Geometry: final body of the model. Coordinates: model frame, mm. A direction names the side the tool comes from. Coordinates: 2 decimals unless noted, no trailing zeros. Order: outer loops, then holes, each group sorted by start corner. A loop starts at its lowest first (then second) coordinate and runs counter-clockwise, first axis right, second up. Notation, with made-up numbers: (50.25, 17.5) -> (86.25, 17.5) arc R22 cw to (86.25, 37.5) -> close; hole circle Ø6 at (-39, 63.25). An arc over 180 degrees is marked (long way). Answer in a Markdown table with one row per item. Add a question column.
1) Section query B-B on x = 2.75. Return the cut outline in (y, z), then the cut area to 3 significant figures.
2) Ray query, line 1 (X direction, y = 3.75, z = 0); line 2 (Z direction, x = -0.75, y = 9); line 3 (X direction, y = 6.5, z = 1.5). Return the intervals inside material, ascending. Write a range as from..to.
3) Contact query for flat-ended pins moving along their axis: P1, Ø3.5, axis at x = -1.5, z = 0.5, coming from the +Y side; P2, Ø6, axis at x = -4.5, y = 6.5, coming from the -Z side; P3, Ø3, axis at y = 3, z = 4.5, coming from the +X side. Output: stop coordinate, or through.
4) Set-up query: faces 4 (the face through (-4.1, 4.93, 4.38)), 5 (the face through (-3.417, 6.056, -0.759)). Return all of +Z, -Z, +X, -X, +Y, -Y with unobstructed straight access to the full face (end or side cutting, diameter ignored); none if empty.
5) Pull-direction query (X, two-part tool) for faces 1 (the face through (0, 2, 0)), 2 (the face through (0, 0, 0)), 3 (the face through (5.699, 5.07, -5.715)); classes: +X half, -X half, draft (parallel to the pull), parting line (faces both ways), or undercut.
6) Section query A-A on y = 3. Return the cut outline in (x, z).
7) Section query D-D on x = 4.5. Return the cut outline in (y, z).
8) Section query C-C on z = -3.25. Return the cut outline in (x, y).
```python
from build123d import *

# Parameters (mm, degrees)
BOSS_EXTRUDE1_DEPTH = 10
SKETCH2_R           = 3.5
CUT_EXTRUDE1_DEPTH  = 8
FILLET1_R           = 1


with BuildPart() as part:
    # Sketch1 → Boss-Extrude1 (new body)
    with BuildSketch(Plane(origin=(0, 0, 0), x_dir=(1, 0, 0), z_dir=(0, 1, 0))):
        with BuildLine():
            Line((0, 6), (6, 6))
            Line((6, 6), (6, 0))
            ThreePointArc((6, 0), (-4.242640687, -4.242640687), (0, 6))
        make_face()
    extrude(amount=BOSS_EXTRUDE1_DEPTH)

    # Sketch2 → Cut-Extrude1 (cut)
    with BuildSketch(Plane(origin=(0, 10, 0), x_dir=(1, 0, 0), z_dir=(0, 1, 0))):
        with Locations(Location((0, 0, 0), (0, 0, 270))):  # turned: the seam where the file's is
            Circle(SKETCH2_R)
    extrude(amount=-CUT_EXTRUDE1_DEPTH, mode=Mode.SUBTRACT)

    # Fillet1
    fillet1_edges = [part.edges().sort_by_distance(p)[0] for p in [
        (6, 5, -6),
    ]]
    fillet(fillet1_edges, radius=FILLET1_R)


solid = part.part
```
Result:
| question | item | result |
|---|---|---|
| 1 | outline | (0, -6) -> (10, -6) -> (10, -2.17) -> (2, -2.17) -> (2, 2.17) -> (10, 2.17) -> (10, 5.33) -> (0, 5.33) -> close |
| 1 | area | 78.7 mm2 |
| 2 | line 1 | -6..-3.5, 3.5..6 |
| 2 | line 2 | -5.95..-3.42, 3.42..5.95 |
| 2 | line 3 | -5.81..-3.16, 3.16..5.81 |
| 3 | P1 | y = 2 |
| 3 | P2 | z = -5.81 |
| 3 | P3 | x = 5.2 |
| 4 | face 4 | +Y, -Y |
| 4 | face 5 | +Y |
| 5 | face 1 | undercut |
| 5 | face 2 | draft |
| 5 | face 3 | +X half |
| 6 | outline | (0, -6) -> (5, -6) arc R1 ccw to (6, -5) -> (6, 0) arc R6 ccw (long way) to start; hole circle Ø7 at (0, 0) |
| 7 | outline | (0, -6) -> (10, -6) -> (10, 3.97) -> (0, 3.97) -> close |
| 8 | outline | (-5.04, 0) -> (6, 0) -> (6, 10) -> (1.3, 10) -> (1.3, 2) -> (-1.3, 2) -> (-1.3, 10) -> (-5.04, 10) -> close |
